```python
from build123d import *

# Parameters (mm, degrees)
BOSS_EXTRUDE1_DEPTH     = 85
SKETCH2_R               = 1.5000000000000007
CUT_EXTRUDE1_DEPTH      = 2.8
CUT_EXTRUDE2_START      = -2.8
SKETCH3_R               = 1.5000000000000007
CUT_EXTRUDE2_DEPTH      = 2.8
CUT_EXTRUDE3_DEPTH      = 5
CUT_EXTRUDE3_DEPTH_BACK = 1
CUT_EXTRUDE4_DEPTH      = 1
CUT_EXTRUDE4_DEPTH_BACK = 1
FILLET1_R               = 2
FILLET2_R               = 1


with BuildPart() as part:
    # Sketch1 → Boss-Extrude1 (new body)
    with BuildSketch(Plane(origin=(0, 0, 0), x_dir=(1, 0, 0), z_dir=(0, 1, 0))):
        with BuildLine():
            Line((-18.500000000000032, 1.9999999999999996), (-21.500000000000068, 1.9999999999999996))
            ThreePointArc((-21.500000000000053, 1.9999999999999463), (-22.499999999999986, -1.91e-15), (-21.50000000000005, -1.9999999999999476))
            Line((-21.500000000000064, -2.0000000000000004), (-18.500000000000036, -2.0000000000000004))
            ThreePointArc((-18.50000000000003, -2.0000000000000226), (-17.763932022500214, -1.1180339887499129), (-17.499999999999993, -6.1e-16))
            ThreePointArc((-17.499999999999993, 0), (-17.763932022500214, 1.1180339887499113), (-18.500000000000025, 2.0000000000000213))
        make_face()
        with BuildLine():
            ThreePointArc((-18.500000000000025, 2.000000000000021), (-20.00000000000005, 2.4999999999999947), (-21.500000000000053, 1.9999999999999463))
            Line((-21.500000000000068, 1.9999999999999996), (-18.500000000000032, 1.9999999999999996))
        make_face()
        with BuildLine():
            Line((-18.500000000000036, -2.0000000000000004), (-21.500000000000064, -2.0000000000000004))
            ThreePointArc((-21.50000000000005, -1.9999999999999476), (-20.000000000000053, -2.4999999999999947), (-18.50000000000003, -2.0000000000000226))
        make_face()
        with BuildLine():
            Line((-21.500000000000068, 1.9999999999999996), (-27.49999999999999, 1.9999999999999996))
            Line((-27.49999999999999, 1.9999999999999996), (-27.49999999999999, -2.0000000000000004))
            Line((-27.49999999999999, -2.0000000000000004), (-21.500000000000064, -2.0000000000000004))
            ThreePointArc((-21.50000000000005, -1.9999999999999476), (-22.499999999999986, -1.91e-15), (-21.500000000000053, 1.9999999999999463))
        make_face()
        with BuildLine():
            Line((18.49999999999991, 1.9999999999999996), (-18.500000000000032, 1.9999999999999996))
            ThreePointArc((-18.500000000000025, 2.0000000000000213), (-17.763932022500214, 1.1180339887499113), (-17.499999999999993, 0))
            ThreePointArc((-17.499999999999993, -6.1e-16), (-17.763932022500214, -1.1180339887499129), (-18.50000000000003, -2.0000000000000226))
            Line((-18.500000000000036, -2.0000000000000004), (18.499999999999925, -2.0000000000000004))
            ThreePointArc((18.499999999999932, -1.9999999999999478), (17.5, -1.91e-15), (18.49999999999993, 1.9999999999999456))
        make_face()
        with BuildLine():
            ThreePointArc((21.49999999999997, 2.00000000000002), (19.99999999999994, 2.4999999999999982), (18.49999999999993, 1.9999999999999456))
            Line((18.49999999999991, 1.9999999999999996), (21.499999999999968, 1.9999999999999996))
        make_face()
        with BuildLine():
            Line((21.499999999999968, 1.9999999999999996), (18.49999999999991, 1.9999999999999996))
            ThreePointArc((18.49999999999993, 1.9999999999999456), (17.5, -1.91e-15), (18.499999999999932, -1.9999999999999478))
            Line((18.49999999999992, -2.0000000000000004), (21.499999999999954, -2.0000000000000004))
            ThreePointArc((21.499999999999964, -2.0000000000000244), (22.23606797749978, -1.1180339887499124), (22.5, -6.1e-16))
            ThreePointArc((22.5, 0), (22.23606797749978, 1.11803398874991), (21.49999999999997, 2.00000000000002))
        make_face()
        with BuildLine():
            Line((21.499999999999954, -2.0000000000000004), (18.49999999999992, -2.0000000000000004))
            ThreePointArc((18.499999999999932, -1.9999999999999478), (19.999999999999936, -2.4999999999999982), (21.499999999999964, -2.0000000000000244))
        make_face()
        with BuildLine():
            Line((27.50000000000001, 1.9999999999999996), (21.499999999999968, 1.9999999999999996))
            ThreePointArc((21.49999999999997, 2.00000000000002), (22.23606797749978, 1.11803398874991), (22.5, 0))
            ThreePointArc((22.5, -6.1e-16), (22.23606797749978, -1.1180339887499124), (21.499999999999964, -2.0000000000000244))
            Line((21.499999999999954, -2.0000000000000004), (27.50000000000001, -2.0000000000000004))
            Line((27.50000000000001, -2.0000000000000004), (27.50000000000001, 1.9999999999999996))
        make_face()
    extrude(amount=BOSS_EXTRUDE1_DEPTH)

    # Sketch2 → Cut-Extrude1 (cut)
    with BuildSketch(Plane(origin=(0, 85, 0), x_dir=(1, 0, 0), z_dir=(0, 1, 0))):
        with Locations(Location((-19.99999999999999, 0, 0), (0, 0, 270))):
            Circle(SKETCH2_R)
        with Locations(Location((20, 0, 0), (0, 0, 270))):
            Circle(SKETCH2_R)
    extrude(amount=-CUT_EXTRUDE1_DEPTH, mode=Mode.SUBTRACT)

    # Sketch3 → Cut-Extrude2 (cut)
    with BuildSketch(Plane.XZ.offset(CUT_EXTRUDE2_START)):
        with Locations(Location((-19.99999999999999, 0, 0), (0, 0, 90))):
            Circle(SKETCH3_R)
        with Locations(Location((20, 0, 0), (0, 0, 90))):
            Circle(SKETCH3_R)
    extrude(amount=CUT_EXTRUDE2_DEPTH, mode=Mode.SUBTRACT)

    # Sketch4 → Cut-Extrude3 (cut, two sides: drawn at the far end of the back side and taken through both)
    with BuildSketch(Plane.XY.offset(2.0000000000000004).offset(-CUT_EXTRUDE3_DEPTH_BACK)):
        Polygon((-27.500000000000018, 80), (27.500000000000007, 80), (27.50000000000001, 4.999999999999997), (-27.50000000000001, 4.999999999999997), align=None)
    extrude(amount=CUT_EXTRUDE3_DEPTH + CUT_EXTRUDE3_DEPTH_BACK, mode=Mode.SUBTRACT)

    # Sketch5 → Cut-Extrude4 (cut, two sides: drawn at the far end of the back side and taken through both)
    with BuildSketch(Plane(origin=(0, 0, -1.9999999999999996), x_dir=(-1, 0, 0), z_dir=(0, 0, -1)).offset(-CUT_EXTRUDE4_DEPTH_BACK)):
        Polygon((-27.49999999999999, 80.00000000000001), (27.49999999999999, 80.00000000000001), (27.49999999999999, 5.0000000000000115), (-27.499999999999982, 5.0000000000000115), align=None)
    extrude(amount=CUT_EXTRUDE4_DEPTH + CUT_EXTRUDE4_DEPTH_BACK, mode=Mode.SUBTRACT)

    # Fillet1
    fillet1_edges = [part.edges().sort_by_distance(p)[0] for p in [
        (-27.49999999999999, 82.5, 2.0000000000000004),
    ]]
    fillet(fillet1_edges, radius=FILLET1_R)
    fillet1_2_edges = [part.edges().sort_by_distance(p)[0] for p in [
        (-27.49999999999999, 2.5000000000000058, -1.9999999999999996),
    ]]
    fillet(fillet1_2_edges, radius=FILLET1_R - 0.0004)  # a hair under: the kernel refuses the full size
    fillet1_3_edges = [part.edges().sort_by_distance(p)[0] for p in [
        (27.50000000000001, 82.5, 2.0000000000000004),
    ]]
    fillet(fillet1_3_edges, radius=FILLET1_R)
    fillet1_4_edges = [part.edges().sort_by_distance(p)[0] for p in [
        (27.50000000000001, 2.5000000000000058, -1.9999999999999996),
    ]]
    fillet(fillet1_4_edges, radius=FILLET1_R - 0.0004)  # a hair under: the kernel refuses the full size

    # Fillet2
    fillet2_edges = [part.edges().sort_by_distance(p)[0] for p in [
        (-19.999999999999986, 80.00000000000001, -2.499999999999992),
        (19.999999999999996, 80.00000000000001, -2.500000000000009),
        (19.999999999999996, 5.0000000000000115, -2.500000000000009),
        (-19.999999999999986, 5.0000000000000115, -2.499999999999992),
        (-5.684e-14, 80.00000000000001, -1.9999999999999996),
        (23.50019999999999, 5.0000000000000115, -1.9999999999999996),
        (-5.329e-14, 5.0000000000000115, -1.9999999999999996),
        (23.500200169244646, 80.00000000000001, -1.9999999999999996),
        (-26.5002999949995, 80.00000000000001, -1.7320466614179624),
        (26.50030014156478, 80.00000000000001, -1.7320465767871778),
        (-23.500200000000024, 5.0000000000000115, -1.9999999999999996),
        (-26.500299994999484, 5.0000000000000115, -1.7320466614179728),
        (26.500299994999494, 5.0000000000000115, -1.7320466614179786),
        (-23.500000000000025, 4.999999999999997, 2.0000000000000004),
        (-26.49999999999999, 5, 1.7320508075688776),
        (26.500000103238282, 5, 1.7320507479642298),
        (23.499999999999982, 80, 2.0000000000000004),
        (-26.499999999999982, 80, 1.7320508075688823),
        (26.50000000000001, 80, 1.732050807568878),
        (-20.000000000000053, 80, 2.4999999999999925),
        (-23.50000000000002, 80, 2.0000000000000004),
        (19.999999999999932, 80, 2.499999999999999),
        (-5.329e-14, 80, 2.0000000000000004),
        (-20.000000000000053, 4.999999999999997, 2.4999999999999925),
        (-5.507e-14, 4.999999999999997, 2.0000000000000004),
        (19.999999999999932, 4.999999999999997, 2.499999999999999),
        (23.500000119209272, 4.999999999999997, 2.0000000000000004),
        (-23.500200000000024, 80.00000000000001, -1.9999999999999996),
    ]]
    fillet(fillet2_edges, radius=FILLET2_R - 0.0001)  # a hair under: the kernel refuses the full size


solid = part.part
```
Verification items for the finished model (mm, model axes). A direction names the side the tool comes from. Give positions to 0.01 mm unless a question says otherwise; leave off trailing zeros. Loops run counter-clockwise (first coordinate to the right, second up) from the corner with the lowest first, then second, coordinate; pieces in that order, holes last. Notation, with made-up numbers: M -4.75,-29 L 49.25,-29 A22 ccw 49.25,-19 Z; hole C -38.5,31.25 d8. An arc over 180 degrees is marked long. One line per question, with ' | ' between items.
Item 1: Tool access check on faces 1 (the face through (21.487, 83.62, -0.195)), 2 (the face through (-24, 2, 2)), 3 (the face through (24, 83, -2)), 4 (the face through (0, 2, 2)), 5 (the face through (20, 2.8, 0)). Record the directions out of +Z, -Z, +X, -X, +Y, -Y that give a thin tool (end or side, any length) a straight path to the whole face; none if there is none.
Completed:
face 1: +Y | face 2: +Z, -X, +Y, -Y | face 3: -Z, +X, +Y, -Y | face 4: +Z, +Y, -Y | face 5: -Y
Item 2: Depth check by flat-ended pin: P1, Ø0.6, axis at x = 7.5, z = -1.5, coming from the -Y side; P2, Ø1.2, axis at x = 23.5, y = 2.5, coming from the -Z side; P3, Ø2, axis at x = 23, y = 2.5, coming from the +Z side; P4, Ø3, axis at x = 22.5, y = 82.5, coming from the +Z side. Enter the tip coordinate at first touch or a pass-through.
Completed:
P1: stops at y = 0 | P2: stops at z = -2 | P3: stops at z = 2 | P4: stops at z = 2.29
Item 3: Draft check along Z on faces 6 (the face through (-20, 82.2, 0)), 7 (the face through (0, 83, -2)), 8 (the face through (0, 85, 0)), 9 (the face through (20, 2, 2.5)). Enter one of: +Z half, -Z half, draft (parallel to the pull), parting line (faces both ways), or undercut.
Completed:
face 6: undercut | face 7: -Z half | face 8: draft | face 9: +Z half
Item 4: Section check B-B, the plane x = 20. Record the cut outline in (y, z), plus the area to 3 significant figures.
Completed:
outline: M 0,-2.5 L 4,-2.5 A1 ccw 5,-1.5 L 5,-1 L 80,-1 L 80,-1.5 A1 ccw 81,-2.5 L 85,-2.5 L 85,-1.5 L 82.2,-1.5 L 82.2,1.5 L 85,1.5 L 85,2.5 L 81,2.5 A1 ccw 80,1.5 L 80,1 L 5,1 L 5,1.5 A1 ccw 4,2.5 L 0,2.5 L 0,1.5 L 2.8,1.5 L 2.8,-1.5 L 0,-1.5 Z | area: 182 mm^2
Item 5: Thickness scan on line 1 (Z direction, x = 20, y = 1.2); line 2 (Y direction, x = 6.5, z = 1.1) (3 decimals); line 3 (Y direction, x = 20.5, z = -0.1). Record the ranges inside material, lowest first. Write a range as [from, to].
Completed:
line 1: z = [-2.5, -1.5], [1.5, 2.5] | line 2: y = [0, 4.995], [80.005, 85] | line 3: y = [2.8, 82.2]
